```python
from build123d import *

# Parameters (mm, degrees)
F0_R     = 22.225
F0_R_2   = 15.875
F1_DEPTH = 12.7
F3_R     = 3.175
F4_DEPTH = 12.7
F5_R     = 1.5875


with BuildPart() as f1:
    # F0 (on Front) → F1 (new body)
    with BuildSketch(Plane.XZ):
        Circle(F0_R)
        Circle(F0_R_2, mode=Mode.SUBTRACT)
    extrude(amount=F1_DEPTH)

    # F3 (on offset) → F4 (cut)
    with BuildSketch(Plane.XY.offset(23.368)):
        with Locations((0, -6.35)):
            Circle(F3_R)
    extrude(amount=-F4_DEPTH, mode=Mode.SUBTRACT)

    # F5
    f5_edges = [f1.edges().sort_by_distance(p)[0] for p in [
        (-22.225, -12.7, 0),
        (-22.225, 0, 0),
    ]]
    fillet(f5_edges, radius=F5_R)


solid = f1.part
```
Can you work these out from the model? Positions are in its coordinate system, mm. Coordinates: 2 decimals unless noted, no trailing zeros. Write each loop counter-clockwise with the first axis right and the second up, starting at its lowest first coordinate (ties: lowest second). Pieces come first, ordered by that corner, then holes. Notation, with made-up numbers: (5.5, -12.75) - (32.5, -12.75) arc R21 ccw to (32.5, 24.25) - close; hole circle Ø7 at (77, 51). An arc over 180 degrees is marked (long way). Return JSON: item names as keys, results as strings.
Q1. Please list where these lines run through material, in increasing order: L1, parallel to Y at x = 0, z = 20.25 (3 decimals); L2, parallel to X at y = -6.35, z = 19.75 (3 decimals); L3, parallel to Z at x = 13, y = -5.5. Write a range as from..to.
Computed values:
{"L1": "y = -12.7..-9.525, -3.175..0", "L2": "x = -10.193..-3.175, 3.175..10.193", "L3": "z = -18.03..-9.11, 9.11..18.03"}
Q2. If we section it at A-A (z = 0): Please give me the cut outline in (x, y) (1 decimal).
Computed values:
{"outline": "(-22.2, -11.1) arc R1.6 ccw to (-20.6, -12.7) - (-15.9, -12.7) - (-15.9, 0) - (-20.6, 0) arc R1.6 ccw to (-22.2, -1.6) - close; (15.9, -12.7) - (20.6, -12.7) arc R1.6 ccw to (22.2, -11.1) - (22.2, -1.6) arc R1.6 ccw to (20.6, 0) - (15.9, 0) - close"}
Q3. If we section it at C-C (y = -6.35): Please give me the cut outline in (x, z) (3 decimals).
Computed values:
{"outline": "(-3.175, 15.554) - (-3.175, 21.997) arc R22.225 ccw (long way) to (3.175, 21.997) - (3.175, 15.554) arc R15.875 cw (long way) to start"}
Q4. Thinking about a two-plate mould opening in Y: for faces 1 (the flat face through (11, 0, -12)), 2 (the cylindrical face through (-0.69, -9.45, 18.94)), 3 (the flat face through (11, -12.7, -12)), which applies, +Y half, -Y half, draft (parallel to the pull), parting line (faces both ways), or undercut?
Computed values:
{"face 1": "+Y half", "face 2": "undercut", "face 3": "-Y half"}
Q5. I'm going to push flat-ended pins straight in: pin 1 Ø5 at (y, z) = (-7.5, 17.5) entering from -X; pin 2 Ø3 at (y, z) = (-6, 6) entering from -X; pin 3 Ø1.5 at (x, y) = (-17, -7.5) entering from -Z. Where does each tip first touch, or does it pass through?
Computed values:
{"pin 1": "stops at x = -16.4", "pin 2": "stops at x = -21.76", "pin 3": "stops at z = -15.16"}
Q6. If we section it at B-B (x = 0): Please give me the cut outline in (y, z) (1 decimal).
Computed values:
{"outline": "(-12.7, -20.6) arc R1.6 ccw to (-11.1, -22.2) - (-1.6, -22.2) arc R1.6 ccw to (0, -20.6) - (0, -15.9) - (-12.7, -15.9) - close; (-12.7, 15.9) - (-9.5, 15.9) - (-9.5, 22.2) - (-11.1, 22.2) arc R1.6 ccw to (-12.7, 20.6) - close; (-3.2, 15.9) - (0, 15.9) - (0, 20.6) arc R1.6 ccw to (-1.6, 22.2) - (-3.2, 22.2) - close"}
